```python
from build123d import *

# Parameters (mm, degrees)
BASE_DEPTH                = 5
SKETCH2_W                 = 130
SKETCH2_H                 = 5
MIDDLE_EXTRUSION_DEPTH    = 15
FANCY_CUTOUT_DEPTH        = 167.602070815
FANCY_CUTOUT_MIDDLE_DEPTH = 168.406690428
OVERALL_FILLETS_R         = 1.25


with BuildPart() as part:
    # Sketch1 → base (new body)
    with BuildSketch(Plane(origin=(0, 0, 0), x_dir=(1, 0, 0), z_dir=(0, 1, 0))):
        Polygon((0, 0), (0, 17.5), (85, 17.5), (85, 2.5), (130, 2.5), (130, -2.5), (165, -2.5), (165, -17.5), (0, -17.5), align=None)
    extrude(amount=BASE_DEPTH)

    # Sketch2 → middle_extrusion (add)
    with BuildSketch(Plane(origin=(0, 5, 0), x_dir=(1, 0, 0), z_dir=(0, 1, 0))):
        with Locations((65, 0)):
            Rectangle(SKETCH2_W, SKETCH2_H)
    extrude(amount=MIDDLE_EXTRUSION_DEPTH)

    # Sketch3 → fancy_cutout (cut, through all)
    with BuildSketch(Plane(origin=(0, 5, 0), x_dir=(1, 0, 0), z_dir=(0, 1, 0))):
        with BuildLine():
            Line((0, -7.5), (0, -2.5))
            ThreePointArc((0, -2.5), (2.5, -5), (0, -7.5))
        make_face()
        with BuildLine():
            Line((0, 2.5), (0, 7.5))
            ThreePointArc((0, 7.5), (2.5, 5), (0, 2.5))
        make_face()
        with BuildLine():
            Line((85, 2.5), (85, 7.5))
            ThreePointArc((85, 7.5), (82.5, 5), (85, 2.5))
        make_face()
    extrude(amount=-FANCY_CUTOUT_DEPTH, mode=Mode.SUBTRACT)

    # Sketch4 → fancy_cutout_middle (cut, through all)
    with BuildSketch(Plane.XY.offset(2.5)):
        with BuildLine():
            Line((0, 5), (0, 10))
            ThreePointArc((0, 10), (2.5, 7.5), (0, 5))
        make_face()
        with BuildLine():
            Line((130, 5), (130, 10))
            ThreePointArc((130, 10), (127.5, 7.5), (130, 5))
        make_face()
    extrude(amount=-FANCY_CUTOUT_MIDDLE_DEPTH, mode=Mode.SUBTRACT)

    # overall_fillets
    overall_fillets_edges = [part.edges().sort_by_distance(p)[0] for p in [
        (0, 2.5, -17.5),
        (85, 2.5, -17.5),
        (165, 2.5, 2.5),
        (165, 2.5, 17.5),
        (0, 2.5, 17.5),
        (130, 20, 0),
        (0, 20, 0),
    ]]
    fillet(overall_fillets_edges, radius=OVERALL_FILLETS_R)


solid = part.part
```
Work out the finished part from the listing and answer in its coordinate system (mm). A direction names the side the tool comes from. Give positions to 0.01 mm unless a question says otherwise; leave off trailing zeros. Order: outer loops, then holes, each group sorted by start corner. A loop starts at its lowest first (then second) coordinate and runs counter-clockwise, first axis right, second up. Notation, with made-up numbers: M -9.5,-12 L -0.5,-12 A11 ccw -0.5,0 Z; hole C 37.25,-30.75 d6. An arc over 180 degrees is marked long. Return JSON: item names as keys, results as strings.
1) A tool of negligible diameter and unlimited length cuts with its end or side. For faces 4 (the flat face through (85, 2, -12)), 5 (the flat face through (43, 5, -10)), 6 (the flat face through (64, 12, 2.5)), 7 (the flat face through (84, 2, 17.5)), from which of +Z, -Z, +X, -X, +Y, -Y can it reach the whole face along a straight path? Write none if from no direction.
Resolved:
{"face 4": "-Z, +X, +Y, -Y", "face 5": "-Z, +X, -X, +Y", "face 6": "+Z, +X, -X, +Y", "face 7": "+Z, +X, -X, +Y, -Y"}
2) Section B-B, the plane z = -14.5 is taken. Write down the section's boundary in (x, y), plus the area to 3 significant figures.
Resolved:
{"outline": "M 0,0 L 85,0 L 85,5 L 0,5 Z", "area": "425 mm^2"}
3) Straight lines are drawn through the part: line 1 along Y through (x, z) = (81, 16.5); line 2 along Z through (x, y) = (15, 5.75); line 3 along X through (y, z) = (4.5, -10). For each, find the intervals that lie inside material, in ascending order. Write a range as [from, to].
Resolved:
{"line 1": "[0, 5]", "line 2": "[-2.5, 2.5]", "line 3": "[0, 85]"}
4) Section A-A, the plane x = 91.5 is taken. Write down the section's boundary in (y, z), plus the area to 3 significant figures.
Resolved:
{"outline": "M 0,-2.5 L 20,-2.5 L 20,2.5 L 5,2.5 L 5,17.5 L 0,17.5 Z", "area": "175 mm^2"}
5) Section C-C, the plane y = 15 is taken. Write down the section's boundary in (x, z), plus the area to 3 significant figures.
Resolved:
{"outline": "M 0,-2.5 L 130,-2.5 L 130,2.5 L 0,2.5 Z", "area": "650 mm^2"}
6) Section D-D, the plane x = 51 is taken. Write down the section's boundary in (y, z).
Resolved:
{"outline": "M 0,-17.5 L 5,-17.5 L 5,-2.5 L 20,-2.5 L 20,2.5 L 5,2.5 L 5,17.5 L 0,17.5 Z"}
7) Each of these flat-tipped pins is pushed along its axis until it touches: pin 1 (7.5 mm diameter, centred on x = 72.5, y = 15, fed in from +Z); pin 2 (1.5 mm diameter, centred on y = 13.5, z = 0, fed in from +X); pin 3 (1.5 mm diameter, centred on x = 141, y = 3.5, fed in from -Z). Where does it stop, or does it pass through?
Resolved:
{"pin 1": "z = 2.5", "pin 2": "x = 130", "pin 3": "z = 2.5"}
8) For a pull along Y with two mould halves and no side action, classify faces 1 (the cylindrical face through (2.5, 7.6, 0)), 2 (the flat face through (84, 5, 10)), 3 (the flat face through (147, 2, 2.5)) as +Y half, -Y half, draft (parallel to the pull), parting line (faces both ways), or undercut.
Resolved:
{"face 1": "undercut", "face 2": "+Y half", "face 3": "draft"}
